Check sheet for the modelled part. Datum: model origin and axes. Units: mm. Give positions to 0.01 mm unless a question says otherwise; leave off trailing zeros. Order: outer loops, then holes, each group sorted by start corner. A loop starts at its lowest first (then second) coordinate and runs counter-clockwise, first axis right, second up.
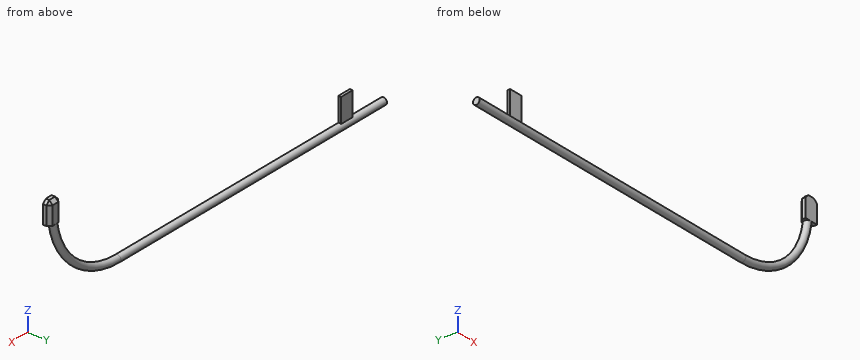
Autodesk Inventor part; units mm, degrees
ref_plane "YZ Plane" through (0, 0, 0) normal (1, 0, 0) x (0, 1, 0)
ref_plane "XZ Plane" through (0, 0, 0) normal (0, 1, 0) x (-1, 0, 0)
ref_plane "XY Plane" through (0, 0, 0) normal (0, 0, 1) x (1, 0, 0)
sketch "Sketch1" plane through (0, 0, 0) normal (1, 0, 0) x (0, 1, 0)
  circle A0 centre (0, 0) radius 3.175
  dimension "d0" = 6.35
sketch "Sketch2" plane through (0, 0, 0) normal (0, 1, 0) x (-1, 0, 0)
  line L0 (0, 0) -> (-292.1, 0)
  arc A0 (-363.942, 71.842) -> (-292.1, 0) centre (-292.1, 71.842) ccw
  line L1 (-292.1, 0) -> (-363.942, 71.842) construction
  line L2 (-292.1, 0) -> (-190.5, 0) construction
  dimension "d1" = 292.1
  dimension "d2" = 101.6
  dimension "d3" = 135
sweep "Sweep1" add profiles "Sketch1" path "Sketch2"
sketch "Sketch3" plane through (0, 0, 0) normal (0, 1, 0) x (-1, 0, 0)
  line L0 (-357.592, 82.002) -> (-370.292, 82.002)
  line L1 (-370.292, 82.002) -> (-370.292, 61.682)
  line L2 (-370.292, 61.682) -> (-357.592, 61.682)
  line L3 (-357.592, 61.682) -> (-357.592, 82.002)
  line L4 (-360.767, 71.842) -> (-367.117, 71.842)
  line L5 (-357.592, 82.002) -> (-370.292, 61.682) construction
  line L6 (-370.292, 82.002) -> (-357.592, 61.682) construction
  point P0 (0, 0)
  point P1 (-363.942, 71.842)
  dimension "d6" = 12.7
  dimension "d7" = 20.32
extrude "Extrusion1" add sketch "Sketch3" along normal mid plane 6.35
chamfer "Chamfer1" distance 3.175 angle 45 5 edges at (370.292, 0, 82.002) (357.592, 0, 82.002) (357.592, 3.175, 71.842) (370.292, 3.175, 71.842) (363.942, 3.175, 82.002)
sketch "Sketch4" plane through (0, 0, 0) normal (0, 1, 0) x (-1, 0, 0)
  line L0 (0, 0) -> (-2.54, 0)
  line L1 (-2.54, 0) -> (-81.28, 0)
  line L2 (-35.56, 25.4) -> (-48.26, 25.4)
  line L3 (-48.26, 25.4) -> (-48.26, -25.4)
  line L4 (-48.26, -25.4) -> (-35.56, -25.4)
  line L5 (-35.56, -25.4) -> (-35.56, 25.4)
  line L6 (-35.56, 25.4) -> (-48.26, -25.4) construction
  line L7 (-48.26, 25.4) -> (-35.56, -25.4) construction
  line L8 (-35.56, 0) -> (-48.26, 0)
  point P0 (-41.91, 0)
  point P1 (-48.26, 0)
  point P2 (-35.56, 0)
  dimension "d13" = 2.54
  dimension "d14" = 78.74
  dimension "d15" = 12.7
  dimension "d16" = 50.8
extrude "Extrusion2" add sketch "Sketch4" along normal mid plane 2.54 contours L1 L3 L2 L5
properties part number "Height adjust(H)"
(1) Gauge pin test, flat ends, axial feed: pin 1 Ø6.5 at (x, z) = (41.5, 18.5) entering from +Y; pin 2 Ø10 at (x, z) = (41, 19) entering from -Y; pin 3 Ø3 at (x, y) = (149.5, -1) entering from +Z (3 decimals). Record the tip position at first contact, or that the pin passes through.
Response values:
pin 1: stops at y = 1.27
pin 2: stops at y = -1.27
pin 3: stops at z = 3.175
(2) Material ranges on L1, parallel to X at y = -1.75, z = 77; L2, parallel to Z at x = 235, y = -0.5; L3, parallel to Y at x = 36.5, z = 13, recorded low to high.
Response values:
L1: x = 357.59 to 370.29
L2: z = -3.14 to 3.14
L3: y = -1.27 to 1.27
(3) Cross-section at A-A on x = 87.5. Enter the section's corners in (y, z) (3 decimals).
Response values:
outline: circle Ø6.35 at (0, 0)
